from build123d import *

# Parameters (mm, degrees)
FILLET_1_R = 1


with BuildPart() as part:
    # Эскиз4 → Повернуть1 (revolve)
    with BuildSketch(Plane(origin=(0, 0, 0), x_dir=(0, 0, -1), z_dir=(1, 0, 0)), mode=Mode.PRIVATE) as revolve_1_sk:
        Polygon((0, 2.8), (0, 7.8), (-4, 11.5), (-4, 10.7), (-0.8, 7.74), (-0.8, 2.8), align=None)
    revolve(revolve_1_sk.sketch.rotate(Axis((0, 0, 0), (0, 0, 1)), 90), axis=Axis((0, 0, 0), (0, 0, 1)))

    # Скругление1
    fillet_1_edges = [part.edges().sort_by_distance(p)[0] for p in [
        (7.74, 0, 0.8),
        (7.8, 0, 0),
    ]]
    fillet(fillet_1_edges, radius=FILLET_1_R)


solid = part.part
Source: CAD feature listing. Evaluate the final solid. Frame: model axes, mm. Coordinates: 2 decimals unless noted, no trailing zeros. Loops run counter-clockwise (first coordinate to the right, second up) from the corner with the lowest first, then second, coordinate; pieces in that order, holes last. Notation, with made-up numbers: (41.5, -8) - (57.5, -8) arc R9 ccw to (57.5, -3) - close; hole circle Ø9 at (9, 0). An arc over 180 degrees is marked (long way). One line per question, with ' | ' between items.
1) Line query: line 1 along Y through (x, z) = (0, 0.3); line 2 along X through (y, z) = (7, 2.85); line 3 along X through (y, z) = (-8, 2.3). Output: solid intervals per line, ascending.
Report:
line 1: y = -8.08 to -2.8, 2.8 to 8.08 | line 2: x = -7.74 to -6.62, 6.62 to 7.74 | line 3: x = -5.88 to -4.39, 4.39 to 5.88
2) Pull-direction query (Y, two-part tool) for faces 1 (the face through (1.8, 8.11, 0.55)), 2 (the face through (-3, 0, 0.8)), 3 (the face through (-3.768, 7.245, 1.261)), 4 (the face through (-8.5, 6.8, 4)); classes: released by +Y, released by -Y, zero draft, split by the parting line, or undercut.
Report:
face 1: split by the parting line | face 2: undercut | face 3: undercut | face 4: zero draft
3) Section C-C, the plane z = 2.4. Return loops of the section in (x, y), then the cut area to 3 significant figures.
Report:
outline: circle Ø20.04 at (0, 0); hole circle Ø18.44 at (0, 0) | area: 48.4 mm²
4) First-contact query: P1, Ø1.5, axis at y = -4, z = 2, coming from the +X side; P2, Ø2, axis at x = 5, z = 1, coming from the +Y side; P3, Ø4.5, axis at x = 2.5, y = -1.5, coming from the +Z side. Flat tips, straight axial feed; report the tip coordinate or a pass-through.
Report:
P1: stops at x = 9.6 | P2: stops at y = 8.4 | P3: stops at z = 0.8
5) Section A-A, the plane x = 0. Return loops of the section in (y, z).
Report:
outline: (-11.5, 4) - (-8.1, 0.32) arc R1 ccw to (-7.36, 0) - (-2.8, 0) - (-2.8, 0.8) - (-7.3, 0.8) arc R1 cw to (-8.04, 1.12) - (-10.7, 4) - close; (2.8, 0) - (7.36, 0) arc R1 ccw to (8.1, 0.32) - (11.5, 4) - (10.7, 4) - (8.04, 1.12) arc R1 cw to (7.3, 0.8) - (2.8, 0.8) - close
